Autodesk Inventor part; units mm, degrees
ref_plane "YZ Plane" through (0, 0, 0) normal (1, 0, 0) x (0, 1, 0)
ref_plane "XZ Plane" through (0, 0, 0) normal (0, 1, 0) x (-1, 0, 0)
ref_plane "XY Plane" through (0, 0, 0) normal (0, 0, 1) x (1, 0, 0)
sketch "Sketch1" plane through (0, 0, 0) normal (0, 0, 1) x (1, 0, 0)
  circle A0 centre (0, 0) radius 25.1
  dimension "d0" = 50.2
extrude "Extrusion1" add sketch "Sketch1" along normal blind 4
sketch "Sketch2" plane through (0, 0, 4) normal (0, 0, 1) x (1, 0, 0)
  line L0 (-15, 3) -> (15, 3)
  line L1 (15, 3) -> (15, -3)
  line L2 (15, -3) -> (-15, -3)
  line L3 (-15, -3) -> (-15, 3)
  point P0 (0, 0)
  point P1 (15, 0)
  point P2 (0, 3)
  dimension "d3" = 30
  dimension "d4" = 6
extrude "Extrusion2" add sketch "Sketch2" along normal blind 5
chamfer "Chamfer1" distance 5 angle 45 2 edges at (15, 0, 9) (-15, 0, 9)
chamfer "Chamfer2" distance 0.5 angle 45 6 edges at (0, -3, 9) (-10.0001, 0, 9) (0, 3, 9) (10.0001, 0, 9) (-25.1, 0, 4) (-25.1, 0, 0)
fillet "Fillet2" radius 2 4 edges at (-12.7501, -3, 6.25) (-12.75, 3, 6.25) (12.75, -3, 6.25) (12.7501, 3, 6.2501)
properties part number "Sensor-Cap" material "ABS Plastic"
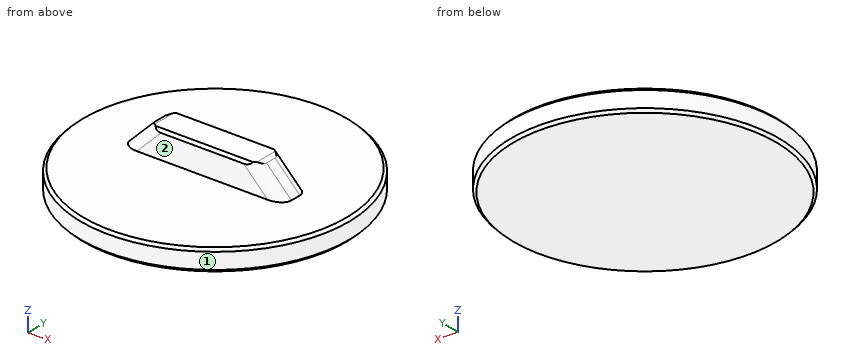
The listing builds one solid part. Answer for the finished solid, in the listing's coordinates (mm). Face numbers are marked on the shaded views. A direction names the side the tool comes from. Round coordinates to 2 decimals unless told otherwise and drop trailing zeros. Write each loop counter-clockwise with the first axis right and the second up, starting at its lowest first coordinate (ties: lowest second). Pieces come first, ordered by that corner, then holes. Notation, with made-up numbers: M 8.5,-6 L 39.5,-6 A22 ccw 39.5,31 Z; hole C 76.5,33 d5. An arc over 180 degrees is marked long. Write each question's results on one line, items separated by ' | '. Start each with the question number.
Item 1: Which of the six approach directions +Z, -Z, +X, -X, +Y, -Y give full straight-line access (tool end or side, diameter ignored) to the marked faces 1 and 2?
Item 2: Straight lines are drawn through the part: probe 1 along Z at (x, y) = (9.5, -16.5); probe 2 along Y at (x, z) = (4.5, 7.5); probe 3 along Y at (x, z) = (-5, 3.5). For each, find the intervals that lie inside material, in ascending order.
Item 3: Find section A-A on x = 0. Write down the section's boundary in (y, z), and give its area (3 significant figures).
Item 4: Given pin 1 Ø1.5 at (y, z) = (2.5, 5) entering from +X; pin 2 Ø3.5 at (x, z) = (1, 6) entering from +Y; pin 3 Ø3 at (y, z) = (-13, 3.5) entering from -X, each flat-ended and moving along its own axis, determine where each tip first touches the part or whether it passes through.
Answer block:
1) face 1: +Z, -Z | face 2: +Z, +X, -X, -Y
2) probe 1: z = 0 to 4 | probe 2: y = -3 to 3 | probe 3: y = -24.6 to 24.6
3) outline: M -25.1,0.5 L -24.6,0 L 24.6,0 L 25.1,0.5 L 25.1,3.5 L 24.6,4 L 3,4 L 3,8.5 L 2.5,9 L -2.5,9 L -3,8.5 L -3,4 L -24.6,4 L -25.1,3.5 Z | area: 230 mm²
4) pin 1: stops at x = 14.18 | pin 2: stops at y = 3 | pin 3: stops at x = -22.31
